Read the model definition and answer for the solid it produces. Units are mm, in the model's axes. Give positions to 0.01 mm unless a question says otherwise; leave off trailing zeros. Write each loop counter-clockwise with the first axis right and the second up, starting at its lowest first coordinate (ties: lowest second). Pieces come first, ordered by that corner, then holes. Notation, with made-up numbers: (-20.75, 49) -> (-13.75, 49) arc R14 cw to (-13.75, 72) -> close; hole circle Ø3 at (-24, 8.5). An arc over 180 degrees is marked (long way). Write item = value, one per line.
Autodesk Inventor part; units mm, degrees
ref_plane "Work Plane3" through (0, 2.5114, 0.6729) normal (0, -0.9659258, -0.258819) x (1, 0, 0)
ref_plane "YZ Plane" through (0, 0, 0) normal (1, 0, 0) x (0, 1, 0)
ref_plane "XZ Plane" through (0, 0, 0) normal (0, 1, 0) x (-1, 0, 0)
sketch "Sketch1" plane through (0, 0, 0) normal (0, 1, 0) x (-1, 0, 0)
  circle A0 centre (0, 0) radius 10
  circle A1 centre (0, 0) radius 3.1
  dimension "d0" = 20
  dimension "d1" = 6.2
extrude "Extrusion1" add sketch "Sketch1" along normal blind 26
ref_plane "Work Plane3" through (0, 2.5114, 0.6729) normal (0, -0.9659258, -0.258819) x (1, 0, 0)
ref_plane "Work Plane2" through (0, 0, 0) normal (0, -0.9659258, -0.258819) x (1, 0, 0)
draft "FaceDraft1" angle 7 pull direction (0, 1, 0) faces at (-9.8705, 17.3333, -1.6041) fixed edges at (10, 0, 0)
sketch "Sketch2" plane through (0, 26, 0) normal (0, 1, 0) x (1, 0, 0)
  point P0 (0, 0)
split "Split1" plane through (0, 2.5114, 0.6729) removes the side toward (0, -0.9659258, -0.258819)
ref_plane "Work Plane1" through (0, 0, 0) normal (0, -1, 0) x (1, 0, 0)
properties part number "cone"
(1) The part is cut by section D-D on y = 7.75. Determine the outline of the cut face in (x, z), plus the area to 3 significant figures.
Checks:
outline = circle Ø18.1 at (0, 0); hole circle Ø6.2 at (0, 0)
area = 227 mm²
(2) Consider L1, parallel to Z at x = 0, y = 14; L2, parallel to X at y = 8, z = 0; L3, parallel to Z at x = -1.75, y = 25. Determine where each line is inside the solid, lowest interval first.
Checks:
L1 = -8.28 to -3.1, 3.1 to 8.28
L2 = -9.02 to -3.1, 3.1 to 9.02
L3 = -6.71 to -2.56, 2.56 to 6.71
(3) The part is cut by section C-C on y = 23.75. Determine the outline of the cut face in (x, z), plus the area to 3 significant figures.
Checks:
outline = circle Ø14.17 at (0, 0); hole circle Ø6.2 at (0, 0)
area = 127 mm²
(4) The part is cut by section A-A on x = 0. Determine the outline of the cut face in (y, z).
Checks:
outline = (0.01, 10) -> (1.86, 3.1) -> (26, 3.1) -> (26, 6.81) -> close; (3.52, -3.1) -> (5.2, -9.36) -> (26, -6.81) -> (26, -3.1) -> close
(5) The part is cut by section B-B on z = 0. Determine the outline of the cut face in (x, y).
Checks:
outline = (-9.67, 2.69) -> (-3.1, 2.69) -> (-3.1, 26) -> (-6.81, 26) -> close; (3.1, 2.69) -> (9.67, 2.69) -> (6.81, 26) -> (3.1, 26) -> close
(6) For a pull along X with two mould halves and no side action, classify faces 1 (the conical face through (1.75, 15.7, 7.88)), 2 (the flat face through (-2.285, 2.066, 2.334)), 3 (the cylindrical face through (0.672, 13.76, 3.026)) as released by +X, released by -X, zero draft, split by the parting line, or undercut.
Checks:
face_1 = split by the parting line
face_2 = zero draft
face_3 = undercut
(7) Given P1, Ø1, axis at y = 5, z = 1.5, coming from the -X side; P2, Ø8, axis at y = 11, z = 1.5, coming from the +X side; P3, Ø8, axis at x = -1, z = -5.5, coming from the -Y side; P4, Ø5, axis at x = 0, z = 0, coming from the -Y side, each flat-ended and moving along its own axis, determine where each tip first touches the part or whether it passes through.
Checks:
P1 = -9.36
P2 = 9.11
P3 = 3.17
P4 = through
